Here's the drawing with two shaded views (mm, measured from the low corner). I have some questions. A direction names the side the tool comes from. Give positions to 0.01 mm unless a question says otherwise; leave off trailing zeros. Write each loop counter-clockwise with the first axis right and the second up, starting at its lowest first coordinate (ties: lowest second). Pieces come first, ordered by that corner, then holes. Notation, with made-up numbers: (86, 38) -> (133, 38) arc R15 ccw to (133, 58) -> close; hole circle Ø1 at (-17, -2.5). An arc over 180 degrees is marked (long way). One line per item, written item: value.
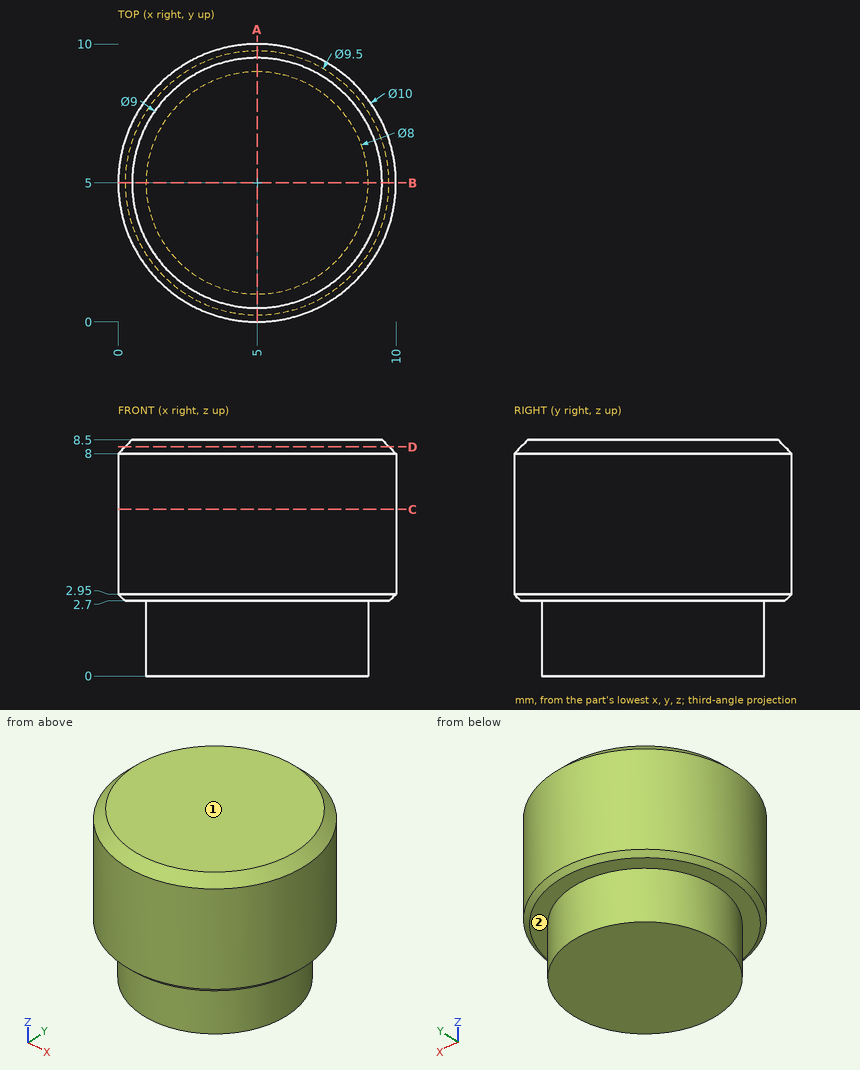
1) I need wall thicknesses on L1, parallel to Z at x = 3, y = 1.5; L2, parallel to X at y = 2.5, z = 4; L3, parallel to Y at x = 9.5, z = 3.5. Which ranges of each line are inside material? Lowest first, please.
Answer list:
L1: z = 2.7 to 8.5
L2: x = 0.67 to 9.33
L3: y = 2.82 to 7.18
2) If we section it at D-D (z = 8.25): Write out the boundary of the cut face in (x, y), and give its area (3 significant figures).
Answer list:
outline: circle Ø9.5 at (5, 5)
area: 70.9 mm^2
3) If we section it at C-C (z = 6): Write out the boundary of the cut face in (x, y).
Answer list:
outline: circle Ø10 at (5, 5)
4) For the marked faces 1 and 2, which set-ups out of +Z, -Z, +X, -X, +Y, -Y let a thin tool reach every point of the face, with its end or its side?
Answer list:
face 1: +Z, +X, -X, +Y, -Y
face 2: -Z
5) Will these pins go through, and if not, where does the flat tip stop? pin 1 (1 mm diameter, centred on x = 2.5, z = 2.5, fed in from +Y); pin 2 (2 mm diameter, centred on y = 1.5, z = 6, fed in from -X).
Answer list:
pin 1: stops at y = 9.45
pin 2: stops at x = 0.67
6) If we section it at A-A (x = 5): Write out the boundary of the cut face in (y, z), and give its area (3 significant figures).
Answer list:
outline: (0, 2.95) -> (0.25, 2.7) -> (1, 2.7) -> (1, 0) -> (9, 0) -> (9, 2.7) -> (9.75, 2.7) -> (10, 2.95) -> (10, 8) -> (9.5, 8.5) -> (0.5, 8.5) -> (0, 8) -> close
area: 79.3 mm^2
